Read the model definition and answer for the solid it produces. Units are mm, in the model's axes. Round coordinates to 2 decimals unless told otherwise and drop trailing zeros. Write each loop counter-clockwise with the first axis right and the second up, starting at its lowest first coordinate (ties: lowest second). Pieces come first, ordered by that corner, then holes. Notation, with made-up numbers: (14.25, 33) -> (63.25, 33) arc R33 ccw to (63.25, 66) -> close; hole circle Ø5 at (71.5, -37.5). An arc over 180 degrees is marked (long way). Return JSON: item names as keys, results as strings. Group by question number.
(1) Straight lines are drawn through the part: line 1 (X direction, y = -1.75, z = 1.75); line 2 (Y direction, x = 100.5, z = -0.25); line 3 (Y direction, x = -237.5, z = -0.5). For each, find the intervals that lie inside material, in ascending order.
(2) A cutting plane is placed at B-B on x = 188.5. Give the vertices of the cut face in (y, z) (3 decimals).
(3) Given pin 1 (2.5 mm diameter, centred on x = -220.5, y = 1.5, fed in from +Z), flat-ended and moving along its own axis, determine where the tip first touches the part or whether it passes through.
```python
from build123d import *

# Parameters (mm, degrees)
F0_R     = 3.175
F1_DEPTH = 260.35
F2_W     = 38.1
F2_H     = 5.08
F3_DEPTH = 12.7
F4_W     = 38.1
F4_H     = 5.08
F5_DEPTH = 12.7


with BuildPart() as f1:
    # F0 (on Right) → F1 (new body, symmetric)
    with BuildSketch(Plane.YZ):
        Circle(F0_R)
    extrude(amount=F1_DEPTH, both=True)

    # F2 (on Front) → F3 (cut, symmetric)
    with BuildSketch(Plane.XZ):
        with Locations((-228.6, 4.1275)):
            Rectangle(F2_W, F2_H)
    extrude(amount=F3_DEPTH, both=True, mode=Mode.SUBTRACT)

    # F4 (on Front) → F5 (cut, symmetric)
    with BuildSketch(Plane.XZ):
        with Locations((-76.2, 4.1275)):
            Rectangle(F4_W, F4_H)
    extrude(amount=F5_DEPTH, both=True, mode=Mode.SUBTRACT)


solid = f1.part
```
Checks:
{
 "1": {"line 1": "x = -260.35 to -247.65, -209.55 to -95.25, -57.15 to 260.35", "line 2": "y = -3.17 to 3.17", "line 3": "y = -3.14 to 3.14"},
 "2": {"outline": "circle Ø6.35 at (0, 0)"},
 "3": {"pin 1": "stops at z = 1.59"}
}
